The model under review builds one solid part; all positions refer to its coordinate system, in mm. A direction names the side the tool comes from. Round coordinates to 2 decimals unless told otherwise and drop trailing zeros. Loops run counter-clockwise (first coordinate to the right, second up) from the corner with the lowest first, then second, coordinate; pieces in that order, holes last. Notation, with made-up numbers: (77.5, 8.25) -> (135.5, 8.25) arc R22 ccw to (135.5, 35.25) -> close; hole circle Ø2 at (5.5, 59.25). An arc over 180 degrees is marked (long way). Use a Markdown table: item, result. Add a question column.
1) Wall thickness on probe 1 along Y at (x, z) = (13, 5.5) (3 decimals); probe 2 along Y at (x, z) = (5, 3): over which ranges is each line inside the solid? List them lowest first.
2) Insertion check: pin 1 (3 mm diameter, centred on y = -19.5, z = 4, fed in from +X) (3 decimals); pin 2 (3 mm diameter, centred on x = 18, z = 4.5, fed in from +Y) (3 decimals); pin 3 (1.9 mm diameter, centred on x = -18.5, z = 3.5, fed in from -Y) (3 decimals). Each pin has a flat end and moves straight along its axis. Give the tip position at first contact, or say it passes through.
3) Consider section B-B on x = 19. Give the boundary of the cut face in (y, z) (3 decimals), plus the area to 3 significant figures.
4) Consider section C-C on y = 7. Give the boundary of the cut face in (x, z).
5) Mouldability with a two-part tool opening along X and no side actions: class faces 1 (the flat face through (0, 0, 6.35)), 2 (the cylindrical face through (-2.245, 9.69, 3.131)), 3 (the cylindrical face through (6.78, 6.69, 3.13)) as released by +X, released by -X, zero draft, split by the parting line, or undercut.
6) For faces 4 (the flat face through (1.905, 17, 3)), 5 (the flat face through (17, -1.905, 3)), 6 (the flat face through (-17, 1.905, 3)), list the 3-axis set-ups (+Z, -Z, +X, -X, +Y, -Y) from which the entire face can be reached by the end or side of a thin tool; tool diameter is ignored.
from build123d import *

# Parameters (mm, degrees)
BOSS_EXTRUDE1_DEPTH = 6.35
SKETCH2_R           = 9.525
BOSS_EXTRUDE2_DEPTH = 6.35
FILLET1_R           = 1.905


with BuildPart() as part:
    # Sketch1 → Boss-Extrude1 (new body)
    with BuildSketch(Plane.XY):
        Polygon((0, 25.4), (1.905, 25.4), (1.905, 1.905), (25.4, 1.905), (25.4, 0), (25.4, -1.905), (1.905, -1.905), (1.905, -25.4), (0, -25.4), (-1.905, -25.4), (-1.905, -1.905), (-25.4, -1.905), (-25.4, 0), (-25.4, 1.905), (-1.905, 1.905), (-1.905, 25.4), align=None)
    extrude(amount=BOSS_EXTRUDE1_DEPTH)

    # Sketch2 → Boss-Extrude2 (add)
    with BuildSketch(Plane.XY):
        Circle(SKETCH2_R)
    extrude(amount=BOSS_EXTRUDE2_DEPTH)

    # Fillet1
    fillet1_edges = [part.edges().sort_by_distance(p)[0] for p in [
        (-9.33255592, -1.905, 3.175),
        (-1.905, -9.33255592, 3.175),
        (-9.33255592, 1.905, 3.175),
        (-1.905, 9.33255592, 3.175),
        (1.905, 9.33255592, 3.175),
        (9.33255592, 1.905, 3.175),
        (9.33255592, -1.905, 3.175),
        (1.905, -9.33255592, 3.175),
        (25.4, 1.905, 3.175),
        (25.4, -1.905, 3.175),
        (1.905, -25.4, 3.175),
        (-1.905, -25.4, 3.175),
        (-25.4, -1.905, 3.175),
        (-25.4, 1.905, 3.175),
        (-1.905, 25.4, 3.175),
        (1.905, 25.4, 3.175),
    ]]
    fillet(fillet1_edges, radius=FILLET1_R - 0.0001)  # a hair under: the kernel refuses the full size


solid = part.part
Result set:
| question | item | result |
|---|---|---|
| 1 | probe 1 | -1.905 to 1.905 |
| 1 | probe 2 | -8.11 to 8.11 |
| 2 | pin 1 | x = 1.905 |
| 2 | pin 2 | y = 1.905 |
| 2 | pin 3 | y = -1.905 |
| 3 | outline | (-1.905, 0) -> (1.905, 0) -> (1.905, 6.35) -> (-1.905, 6.35) -> close |
| 3 | area | 24.2 mm2 |
| 4 | outline | (-6.46, 0) -> (6.46, 0) -> (6.46, 6.35) -> (-6.46, 6.35) -> close |
| 5 | face 1 | zero draft |
| 5 | face 2 | released by -X |
| 5 | face 3 | released by +X |
| 6 | face 4 | +Z, -Z, +X, +Y |
| 6 | face 5 | +Z, -Z, +X, -Y |
| 6 | face 6 | +Z, -Z, -X, +Y |
